Could you check a few things on this drawing? It's one solid part, dimensions in mm from its lowest x, y, z. Give positions to 0.01 mm unless a question says otherwise; leave off trailing zeros. Loops run counter-clockwise (first coordinate to the right, second up) from the corner with the lowest first, then second, coordinate; pieces in that order, holes last. Notation, with made-up numbers: (71.25, -29.75) - (117.25, -29.75) arc R21 ccw to (117.25, -24.75) - close; hole circle Ø5 at (62.25, 79.5). An arc over 180 degrees is marked (long way). One line per item, written item: value. Start each with the question number.
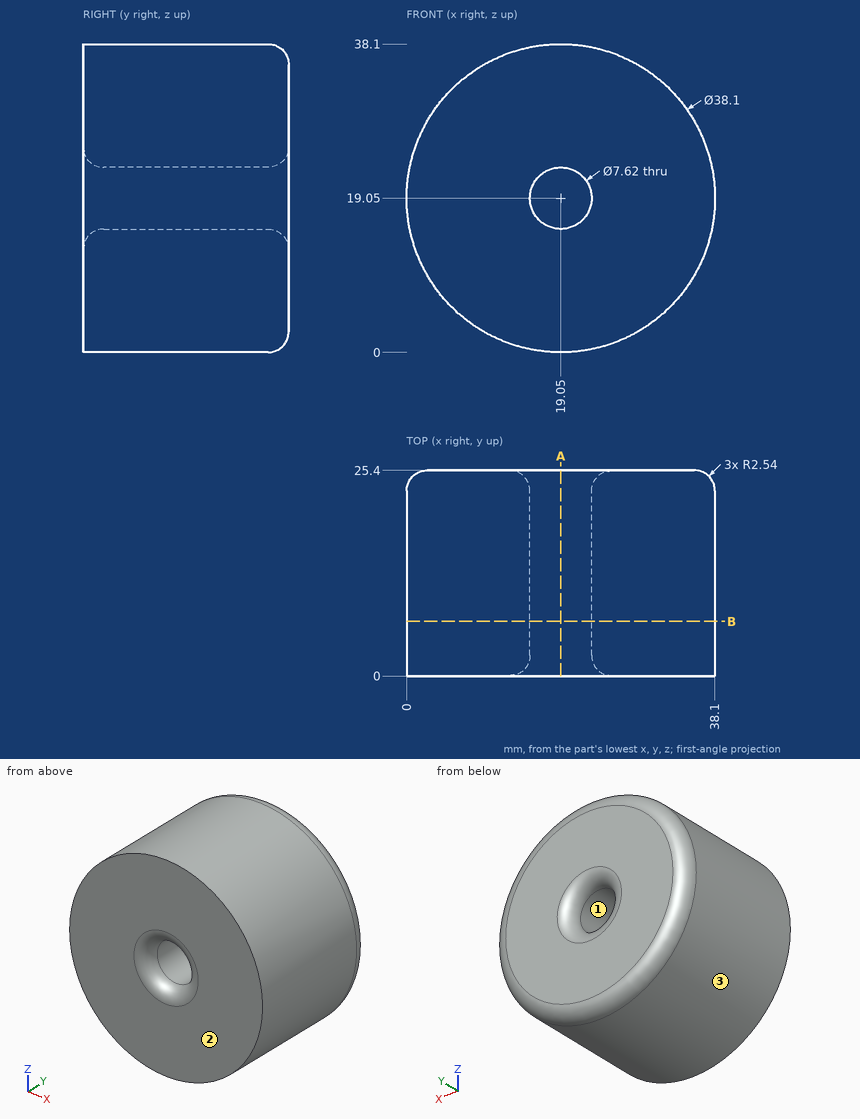
(1) If we section it at A-A on x = 19.05: List the corners of the cut face in (y, z) for me.
(2) If we mould it in two halves opening along X, with no side actions, what happens to the marked faces 1, 2 and 3? For each: pulls with the +X half, pulls with the -X half, needs draft (parallel to the pull), parting line crosses it, or undercut.
(3) Will these pins go through, and if not, where does the flat tip stop? pin 1 (3 mm diameter, centred on x = 22.5, y = 17.5, fed in from -Z); pin 2 (5 mm diameter, centred on y = 9, z = 15, fed in from +X); pin 3 (9 mm diameter, centred on x = 19.05, z = 19.05, fed in from -Y); pin 4 (1.5 mm diameter, centred on x = 29.5, z = 16.5, fed in from -Y).
(4) Please list where these lines run through material, in increasing order: probe 1 along X at (y, z) = (7.5, 19.05); probe 2 along Z at (x, y) = (20, 20.5); probe 3 along X at (y, z) = (2.75, 30). Write a range as from..to.
(5) If we section it at B-B on y = 6.75: List the corners of the cut face in (x, z) for me, plus the area to 3 significant figures.
Found:
1. outline: (0, 0) - (22.86, 0) arc R2.54 ccw to (25.4, 2.54) - (25.4, 12.7) arc R2.54 ccw to (22.86, 15.24) - (2.54, 15.24) arc R2.54 ccw to (0, 12.7) - close; (0, 25.4) arc R2.54 ccw to (2.54, 22.86) - (22.86, 22.86) arc R2.54 ccw to (25.4, 25.4) - (25.4, 35.56) arc R2.54 ccw to (22.86, 38.1) - (0, 38.1) - close
2. face 1: undercut
2. face 2: needs draft
2. face 3: parting line crosses it
3. pin 1: z = 0.1
3. pin 2: x = 38.04
3. pin 3: y = 0.8
3. pin 4: y = 0
4. probe 1: 0..15.24, 22.86..38.1
4. probe 2: 0.02..15.36, 22.74..38.08
4. probe 3: 3.46..34.64
5. outline: circle Ø38.1 at (19.05, 19.05); hole circle Ø7.62 at (19.05, 19.05)
5. area: 1,090 mm^2
